```python
from build123d import *

# Parameters (mm, degrees)
BOSS_EXTRUDE1_DEPTH      = 6
BOSS_EXTRUDE1_2_DEPTH    = 6
SKETCH2_R                = 5.838683498871983
BOSS_EXTRUDE2_DEPTH      = 6
CUT_EXTRUDE1_DEPTH       = 14.695520617658893
CUT_EXTRUDE1_DEPTH_BACK  = 14.695520617658893
SKETCH4_R                = 1.5000000000000004
SKETCH5_W                = 10
SKETCH5_H                = 5.878381978264198
CUT_EXTRUDE2_DEPTH       = 6
CUT_EXTRUDE19_DEPTH      = 11.206882481933452
CUT_EXTRUDE19_DEPTH_BACK = 11.206882481933452
SKETCH31_R               = 1.1
SKETCH33_W               = 5.1
SKETCH33_H               = 1.7000000000000002
CUT_EXTRUDE20_DEPTH      = 6.03
BOSS_EXTRUDE3_DEPTH      = 0.7
BOSS_EXTRUDE4_DEPTH      = 1.7
CUT_EXTRUDE21_START      = 0.7
SKETCH36_R               = 3.05
CUT_EXTRUDE21_DEPTH      = 0.7
SKETCH37_R               = 2.05
CUT_EXTRUDE22_DEPTH      = 6.03
FILLET1_R                = 3.015
FILLET2_R                = 2.5
CUT_EXTRUDE23_DEPTH      = 4.82
CUT_EXTRUDE23_DEPTH_BACK = 4.82
SKETCH39_R               = 2.5500000000000003
CUT_EXTRUDE24_DEPTH      = 3.16
CUT_EXTRUDE24_DEPTH_BACK = 3.16
SKETCH40_R               = 3.025
CHAMFER1_START           = -3.16
CHAMFER1_DEPTH           = 6.32


with BuildPart() as part:
    # Sketch1 → Boss-Extrude1 (new body)
    with BuildSketch(Plane.XY):
        Polygon((-2.4999999999999982, -3.015), (-2.499999999999999, 3.015), (-4.999999999999999, 3.015), (-4.999999999999999, -3.015), align=None)
    extrude(amount=BOSS_EXTRUDE1_DEPTH)



with BuildPart() as body_2:
    # Sketch1 → Boss-Extrude1 2 (new body)
    with BuildSketch(Plane.XY):
        Polygon((5.000000000000001, 3.015), (2.500000000000001, 3.015), (2.5000000000000018, -3.015), (5.000000000000001, -3.015), align=None)
    extrude(amount=BOSS_EXTRUDE1_2_DEPTH)


with BuildPart() as part_1:
    add(part.part)

    add(body_2.part)  # Boss-Extrude2 merges body 2
    # Sketch2 → Boss-Extrude2 (add)
    with BuildSketch(Plane(origin=(0, 0, 0), x_dir=(-1, 0, 0), z_dir=(0, 0, -1))):
        with Locations(Location((0, 0, 0), (0, 0, 148.91002298))):
            Circle(SKETCH2_R)
    extrude(amount=BOSS_EXTRUDE2_DEPTH)

    # Sketch4 → Cut-Extrude1 (cut, two sides: drawn at the far end of the back side and taken through both)
    with BuildSketch(Plane.ZY.offset(4.999999999999999).offset(-CUT_EXTRUDE1_DEPTH_BACK)):
        with Locations((3, 0)):
            Circle(SKETCH4_R)
    extrude(amount=CUT_EXTRUDE1_DEPTH + CUT_EXTRUDE1_DEPTH_BACK, mode=Mode.SUBTRACT)

    # Sketch5 → Cut-Extrude2 (cut)
    with BuildSketch(Plane.XY):
        with Locations((4.4e-16, -5.954190989132099)):
            Rectangle(SKETCH5_W, SKETCH5_H)
    extrude(amount=-CUT_EXTRUDE2_DEPTH, mode=Mode.SUBTRACT)

    # Sketch31 → Cut-Extrude19 (cut, two sides: drawn at the far end of the back side and taken through both)
    with BuildSketch(Plane.XY.offset(-CUT_EXTRUDE19_DEPTH_BACK)):
        Circle(SKETCH31_R)
    extrude(amount=CUT_EXTRUDE19_DEPTH + CUT_EXTRUDE19_DEPTH_BACK, mode=Mode.SUBTRACT)

    # Sketch33 → Cut-Extrude20 (cut)
    with BuildSketch(Plane(origin=(0, -3.015, 0), x_dir=(-1, 0, 0), z_dir=(0, -1, 0))):
        with Locations((-8.9e-16, 5.15)):
            Rectangle(SKETCH33_W, SKETCH33_H)
        Polygon((3.0500000000000056, 4.299999999999999), (2.549999999999999, 4.299999999999999), (-2.5500000000000007, 4.3), (-3.049999999999994, 4.299999999999999), (-3.049999999999994, 3.599999999999999), (3.0500000000000056, 3.6), align=None)
    extrude(amount=-CUT_EXTRUDE20_DEPTH, mode=Mode.SUBTRACT)

    # Sketch34 → Boss-Extrude3 (add)
    with BuildSketch(Plane(origin=(5.1e-16, 0, -3.5999999999999996), x_dir=(-1, 0, -1.4e-16), z_dir=(1.4e-16, 0, -1))):
        with BuildLine():
            ThreePointArc((0.4607331114646439, 3.0150000000000117), (2.313842690198183, 1.9871165051441753), (3.049999999999994, 0))
            Line((3.049999999999994, 0), (3.050000000000006, 3.015))
            Line((3.050000000000006, 3.015), (0.46073311146464313, 3.015))
        make_face()
        with BuildLine():
            Line((-3.0499999999999936, 3.015), (-3.049999999999994, 0))
            ThreePointArc((-3.049999999999994, 3.7e-16), (-2.313842690198182, 1.987116505144176), (-0.46073311146464346, 3.0150000000000117))
            Line((-0.4607331114646427, 3.015), (-3.0499999999999936, 3.015))
        make_face()
    extrude(amount=BOSS_EXTRUDE3_DEPTH)

    # Sketch35 → Boss-Extrude4 (add)
    with BuildSketch(Plane(origin=(0, 0, -6), x_dir=(-1, 0, 0), z_dir=(0, 0, -1))):
        with BuildLine():
            ThreePointArc((-2.550000000000001, -8.2e-16), (-4.1e-16, 2.550000000000001), (2.550000000000001, 0))
            Line((2.5500000000000007, 0), (2.549999999999999, 3.015))
            Line((2.549999999999999, 3.015), (-2.5500000000000007, 3.015))
            Line((-2.5500000000000007, 3.015), (-2.5500000000000007, 0))
        make_face()
    extrude(amount=-BOSS_EXTRUDE4_DEPTH)

    # Sketch36 → Cut-Extrude21 (cut)
    with BuildSketch(Plane.XY.offset(-4.299999999999999).offset(CUT_EXTRUDE21_START)):
        Circle(SKETCH36_R)
    extrude(amount=-CUT_EXTRUDE21_DEPTH, mode=Mode.SUBTRACT)

    # Sketch37 → Cut-Extrude22 (cut)
    with BuildSketch(Plane(origin=(5.1e-16, 0, -3.5999999999999996), x_dir=(-1, 0, -1.4e-16), z_dir=(1.4e-16, 0, -1))):
        Circle(SKETCH37_R)
    extrude(amount=-CUT_EXTRUDE22_DEPTH, mode=Mode.SUBTRACT)

    # Fillet1
    fillet1_edges = [part_1.edges().sort_by_distance(p)[0] for p in [
        (-3.749999999999999, 3.015, 6),
        (-3.7499999999999987, -3.015, 6),
        (3.7500000000000013, -3.015, 6),
        (3.750000000000001, 3.015, 6),
    ]]
    fillet(fillet1_edges, radius=FILLET1_R - 0.0001)  # a hair under: the kernel refuses the full size

    # Fillet2
    # the kernel refuses this fillet: 2.5 mm, written as the material it adds along each edge
    with BuildSketch(Plane(origin=(5.000000000000001, 3.015, 0), x_dir=(0, 1, 0), z_dir=(-1, 0, 0))) as fillet2_piece_1_section:
        with BuildLine():
            CenterArc((FILLET2_R, -FILLET2_R), FILLET2_R, 90, 90)
            Line((-4.4e-16, -FILLET2_R), (0, 0))
            Line((0, 0), (FILLET2_R, 0))
        make_face()
    fillet2_piece_1 = extrude(amount=2.5, mode=Mode.PRIVATE)
    fillet2_piece_1 = fillet2_piece_1 & Plane(origin=(0, 0, 0), x_dir=(0.8563574307404789, 0.5163835307361826, 0), z_dir=(0, 0, 1)) * Cylinder(5.838683498871983, 15, mode=Mode.PRIVATE)
    add(fillet2_piece_1)
    with BuildSketch(Plane(origin=(5.000000000000001, 3.015, 0), x_dir=(0, 1, 0), z_dir=(-1, 0, 0))) as fillet2_piece_2_section:
        with BuildLine():
            CenterArc((FILLET2_R, -FILLET2_R), FILLET2_R, 90, 90)
            Line((-4.4e-16, -FILLET2_R), (0, 0))
            Line((0, 0), (FILLET2_R, 0))
        make_face()
    fillet2_piece_2 = extrude(amount=8.749999999999998, mode=Mode.PRIVATE)
    fillet2_piece_2 = fillet2_piece_2 & Plane(origin=(0, 0, 0), x_dir=(0.8563574307404789, 0.5163835307361826, 0), z_dir=(0, 0, 1)) * Cylinder(5.838683498871983, 28, mode=Mode.PRIVATE)
    fillet2_piece_2 = split(fillet2_piece_2, bisect_by=Plane(origin=(-2.499999999999999, 3.0149999999999992, 0), z_dir=(-1, -1.5e-16, 0)), keep=Keep.TOP, mode=Mode.PRIVATE)
    add(fillet2_piece_2)
    with BuildSketch(Plane(origin=(3.75, 3.015, 0), x_dir=(0, 1, 0), z_dir=(-1, 0, 0))) as fillet2_piece_3_section:
        with BuildLine():
            CenterArc((FILLET2_R, -FILLET2_R), FILLET2_R, 90, 90)
            Line((-4.4e-16, -FILLET2_R), (0, 0))
            Line((0, 0), (FILLET2_R, 0))
        make_face()
    fillet2_piece_3 = extrude(amount=8.75, mode=Mode.PRIVATE)
    fillet2_piece_3 = fillet2_piece_3 & Plane(origin=(0, 0, 0), x_dir=(0.8563574307404789, 0.5163835307361826, 0), z_dir=(0, 0, 1)) * Cylinder(5.838683498871983, 28, mode=Mode.PRIVATE)
    fillet2_piece_3 = split(fillet2_piece_3, bisect_by=Plane(origin=(2.500000000000001, 3.015, 0), z_dir=(1, 1.5e-16, 0)), keep=Keep.TOP, mode=Mode.PRIVATE)
    add(fillet2_piece_3)
    with BuildSketch(Plane(origin=(-2.499999999999999, 3.015, 0), x_dir=(0, 1, 0), z_dir=(-1, 0, 0))) as fillet2_piece_4_section:
        with BuildLine():
            CenterArc((FILLET2_R, -FILLET2_R), FILLET2_R, 90, 90)
            Line((-4.4e-16, -FILLET2_R), (0, 0))
            Line((0, 0), (FILLET2_R, 0))
        make_face()
    fillet2_piece_4 = extrude(amount=2.5, mode=Mode.PRIVATE)
    fillet2_piece_4 = fillet2_piece_4 & Plane(origin=(0, 0, 0), x_dir=(0.8563574307404789, 0.5163835307361826, 0), z_dir=(0, 0, 1)) * Cylinder(5.838683498871983, 15, mode=Mode.PRIVATE)
    add(fillet2_piece_4)

    # Sketch39 → Cut-Extrude23 (cut, two sides: drawn at the far end of the back side and taken through both)
    with BuildSketch(Plane(origin=(0, 0, 0), x_dir=(0, 0, -1), z_dir=(1, 0, 0)).offset(-CUT_EXTRUDE23_DEPTH_BACK)):
        with Locations((-3, 0)):
            Circle(SKETCH39_R)
    extrude(amount=CUT_EXTRUDE23_DEPTH + CUT_EXTRUDE23_DEPTH_BACK, mode=Mode.SUBTRACT)

    # Sketch40 → Cut-Extrude24 (cut, two sides: drawn at the far end of the back side and taken through both)
    with BuildSketch(Plane(origin=(0, 0, 0), x_dir=(0, 0, -1), z_dir=(1, 0, 0)).offset(-CUT_EXTRUDE24_DEPTH_BACK)):
        with Locations((-3, 0)):
            Circle(SKETCH40_R)
    extrude(amount=CUT_EXTRUDE24_DEPTH + CUT_EXTRUDE24_DEPTH_BACK, mode=Mode.SUBTRACT)

    # Chamfer1: read off the stored shape, not the designer's step
    # Chamfer1 outline → Chamfer1 (cut)
    with BuildSketch(Plane.YZ.offset(CHAMFER1_START)):
        with BuildLine():
            ThreePointArc((3.015, 2.754235885), (2.988173778, 2.529423252), (2.944608274, 2.307246717))
            Line((2.944608274, 2.307246717), (3.023955784, 2.288579294))
            ThreePointArc((3.023955784, 2.288579294), (3.01723995, 2.394194848), (3.015, 2.5))
            Line((3.015, 2.5), (3.015, 2.754235885))
        make_face()
        with BuildLine():
            Line((-3.015, 1.754235885), (-2.756573375, 1.754235885))
            ThreePointArc((-2.756573375, 1.754235885), (-2.928782137, 2.243124716), (-3.015, 2.754235885))
            Line((-3.015, 2.754235885), (-3.015, 1.754235885))
        make_face()
    extrude(amount=CHAMFER1_DEPTH, mode=Mode.SUBTRACT)


solid = part_1.part
```
Model file for the job. Use its own axes, mm. A direction names the side the tool comes from. Coordinates: 2 decimals unless noted, no trailing zeros. Order: outer loops, then holes, each group sorted by start corner. A loop starts at its lowest first (then second) coordinate and runs counter-clockwise, first axis right, second up. Notation, with made-up numbers: (4, 17) - (28, 17) arc R4 cw to (28, 23) - close; hole circle Ø10 at (2, 21). An arc over 180 degrees is marked (long way). Return JSON: item names as keys, results as strings. Group by question number.
1) Probe line 1 (Z direction, x = 4.9, y = 0); line 2 (X direction, y = 0.5, z = 5); line 3 (Y direction, x = 4.4, z = 3). List the from-to ranges inside material, lowest first. Write a range as from..to.
2) Saw through at B-B, the plane z = 2.75. Write the cut outline in (x, y) (3 decimals), plus the area to 3 significant figures.
3) Flat gauge pins, fed straight in: P1, Ø4, axis at x = -1, y = 3, coming from the +Z side; P2, Ø4, axis at y = 0, z = 3, coming from the +X side; P3, Ø0.5, axis at y = -2, z = -5, coming from the -X side; P4, Ø2.5, axis at y = 0, z = 3, coming from the +X side. Where does each tip first touch, or does it go through?
4) Mould opens along Y. For faces 1 (the flat face through (-2.55, -2, -5)), 2 (the cylindrical face through (-4.09, 2.11, 5.14)), 3 (the cylindrical face through (-4.002, 0.112, 5.548)) say: released by +Y, released by -Y, zero draft, split by the parting line, or undercut.
5) Tool access for faces 4 (the flat face through (-5, 0, 1)), 5 (the cylindrical face through (0.07, 3.05, -3.95)), 6 (the flat face through (2.5, 3, 1)): list every direction of +Z, -Z, +X, -X, +Y, -Y with a clear straight run to the whole face (end or side of a thin tool).
6) Saw through at A-A, the plane x = 0. Write the cut outline in (y, z) (3 decimals).
Values found:
{
 "1": {"line 1": "z = -6..1.5, 4.5..6", "line 2": "x = -5..-4.82, 4.82..5", "line 3": "y = -3.01..-2.55, 2.55..3.01"},
 "2": {"outline": "(-5, -3.015) - (-3.16, -3.015) - (-3.16, -2.538) - (-4.82, -2.538) - (-4.82, -1.479) - (-5, -1.479) - close; (-5, 1.479) - (-4.82, 1.479) - (-4.82, 2.538) - (-3.16, 2.538) - (-3.16, 3.015) - (-5, 3.015) - close; (3.16, -3.015) - (5, -3.015) - (5, -1.479) - (4.82, -1.479) - (4.82, -2.538) - (3.16, -2.538) - close; (3.16, 2.538) - (4.82, 2.538) - (4.82, 1.479) - (5, 1.479) - (5, 3.015) - (3.16, 3.015) - close", "area": "4.28 mm²"},
 "3": {"P1": "stops at z = 2.31", "P2": "stops at x = 5", "P3": "stops at x = -5.57", "P4": "passes through"},
 "4": {"face 1": "zero draft", "face 2": "released by +Y", "face 3": "undercut"},
 "5": {"face 4": "+Z, -X, +Y, -Y", "face 5": "-Y", "face 6": "+Z, +Y, -Y"},
 "6": {"outline": "(-3.015, -3.6) - (-2.05, -3.6) - (-2.05, 0) - (-3.015, 0) - close; (2.05, -3.6) - (3.05, -3.6) - (3.05, -4.3) - (2.55, -4.3) - (2.55, -6) - (5.839, -6) - (5.839, 0) - (2.05, 0) - close"}
}
